The model under review builds one solid part; all positions refer to its coordinate system, in mm. A direction names the side the tool comes from. Give positions to 0.01 mm unless a question says otherwise; leave off trailing zeros. Order: outer loops, then holes, each group sorted by start corner. A loop starts at its lowest first (then second) coordinate and runs counter-clockwise, first axis right, second up.
```python
from build123d import *

# Parameters (mm, degrees)
BOSS_EXTRUDE1_DEPTH = 4.7752
SKETCH4_W           = 4.7752
SKETCH4_H           = 4.7752
CUT_EXTRUDE1_DEPTH  = 5.7752


with BuildPart() as part:
    # Sketch1 → Boss-Extrude1 (new body)
    with BuildSketch(Plane.XY):
        with BuildLine():
            Line((-4.5504, 44.7752), (-4.5504, 0.2248))
            ThreePointArc((-4.5504, 0.2248), (-3.085933906, -3.310733906), (0.4496, -4.7752))
            Line((0.4496, -4.7752), (15.4496, -4.7752))
            ThreePointArc((15.4496, -4.7752), (18.985133906, -3.310733906), (20.4496, 0.2248))
            Line((20.4496, 0.2248), (20.4496, 44.7752))
            ThreePointArc((20.4496, 44.7752), (18.985133906, 48.310733906), (15.4496, 49.7752))
            Line((15.4496, 49.7752), (0.4496, 49.7752))
            ThreePointArc((0.4496, 49.7752), (-3.085933906, 48.310733906), (-4.5504, 44.7752))
        make_face()
    extrude(amount=BOSS_EXTRUDE1_DEPTH)

    # Sketch4 → Cut-Extrude1 (cut, through all)
    with BuildSketch(Plane.XY.offset(4.7752)):
        with Locations((-2.1628, 22.5)):
            Rectangle(SKETCH4_W, SKETCH4_H)
    extrude(amount=-CUT_EXTRUDE1_DEPTH, mode=Mode.SUBTRACT)


solid = part.part
```
Item 1: Take a section at B-B (z = 1.7). Give the boundary of the cut face in (x, y).
Values found:
outline: (-4.55, 0.22) arc R5 ccw to (0.45, -4.78) - (15.45, -4.78) arc R5 ccw to (20.45, 0.22) - (20.45, 44.78) arc R5 ccw to (15.45, 49.78) - (0.45, 49.78) arc R5 ccw to (-4.55, 44.78) - (-4.55, 24.89) - (0.22, 24.89) - (0.22, 20.11) - (-4.55, 20.11) - close
Item 2: For faces 1 (the cylindrical face through (18.946, -3.349, 2.354)), 2 (the flat face through (-2, 24.888, 2)), list the 3-axis set-ups (+Z, -Z, +X, -X, +Y, -Y) from which the entire face can be reached by the end or side of a thin tool; tool diameter is ignored.
Values found:
face 1: +Z, -Z, +X, -Y
face 2: +Z, -Z, -X
Item 3: Take a section at A-A (x = -0.5). Give the boundary of the cut face in (y, z).
Values found:
outline: (-4.68, 0) - (20.11, 0) - (20.11, 4.78) - (-4.68, 4.78) - close; (24.89, 0) - (49.68, 0) - (49.68, 4.78) - (24.89, 4.78) - close
Item 4: Clearance check with flat-ended pins moving along their axes: pin 1 Ø1.4 at (y, z) = (23.5, 2.5) entering from -X; pin 2 Ø2.5 at (x, z) = (-1.5, 1.5) entering from +Y; pin 3 Ø2.5 at (x, z) = (-2, 1.5) entering from -Y. State where each tip first meets the part, or that it passes through.
Values found:
pin 1: stops at x = 0.22
pin 2: stops at y = 49.73
pin 3: stops at y = -4.63
Item 5: For line 1 (Y direction, x = 16.75, z = 3.4); line 2 (Y direction, x = -1.25, z = 4.1); line 3 (Y direction, x = 18.75, z = 0.8), list the stretches that pass through material, from the lowest coordinate up.
Values found:
line 1: y = -4.6 to 49.6
line 2: y = -4.48 to 20.11, 24.89 to 49.48
line 3: y = -3.53 to 48.53
Item 6: Draft analysis for pull direction Y (two halves, no side actions). For faces 3 (the cylindrical face through (19.024, 48.272, 2.354)), 4 (the flat face through (0.225, 22, 2)), 5 (the flat face through (8, 23, 0)), 6 (the flat face through (-2, 20.112, 2)), state which applies: released by +Y, released by -Y, zero draft, split by the parting line, or undercut.
Values found:
face 3: released by +Y
face 4: undercut
face 5: zero draft
face 6: undercut
Item 7: Take a section at C-C (y = 24). Give the boundary of the cut face in (x, z), and give its area (3 significant figures).
Values found:
outline: (0.22, 0) - (20.45, 0) - (20.45, 4.78) - (0.22, 4.78) - close
area: 96.6 mm2
